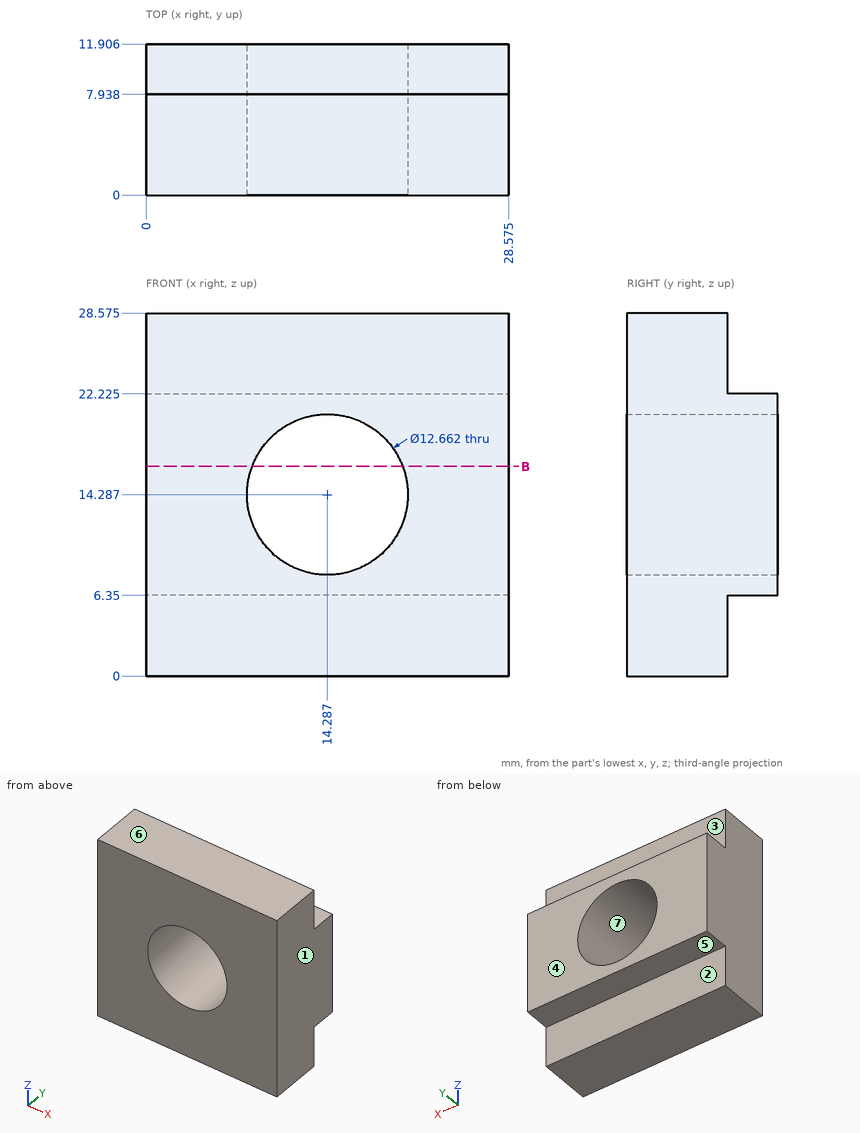
Can you work these out from the drawing? Everything is in mm from the part's minimum corner. A direction names the side the tool comes from. Give positions to 0.01 mm unless a question says otherwise; leave off trailing zeros. Order: outer loops, then holes, each group sorted by start corner. A loop starts at its lowest first (then second) coordinate and runs counter-clockwise, first axis right, second up. Notation, with made-up numbers: M 65.5,50.5 L 71.5,50.5 A30 ccw 71.5,87.5 Z; hole C 87,24.25 d4. An arc over 180 degrees is marked long. Use a Markdown table: item, result. Add a question column.
1. I need wall thicknesses on probe 1 along Y at (x, z) = (11.5, 2.5); probe 2 along X at (y, z) = (5.75, 12.5) (1 decimal); probe 3 along Z at (x, y) = (13.25, 6) (1 decimal). Which ranges of each line are inside material? Lowest first, please. Write a range as from..to.
2. If we mould it in two halves opening along Z, with no side actions, what happens to the marked faces 4, 5, 6 and 7? For each: +Z half, -Z half, draft (parallel to the pull), parting line (faces both ways), or undercut.
3. On a 3-axis mill with a long thin cutter (end or side, diameter ignored), from which of +Z, -Z, +X, -X, +Y, -Y can I reach the whole of each face in a straight line? I mean the marked faces 1, 2 and 3. Say none if no direction works.
4. For pin 1 Ø3 at (x, y) = (13, 10) entering from -Z; pin 2 Ø7 at (x, z) = (9, 2) entering from +Y; pin 3 Ø7.5 at (x, z) = (14.29, 14.29) entering from -Y, each with a flat end and sliding along its axis, tell me the tip position at first contact or that it passes through.
5. Suppose I cut it at B-B (z = 16.5). List the corners of the cut face in (x, y) for me (1 decimal).
Results list:
| question | item | result |
|---|---|---|
| 1 | probe 1 | y = 0..7.94 |
| 1 | probe 2 | x = 0..8.2, 20.4..28.6 |
| 1 | probe 3 | z = 0..8, 20.5..28.6 |
| 2 | face 4 | draft |
| 2 | face 5 | -Z half |
| 2 | face 6 | +Z half |
| 2 | face 7 | undercut |
| 3 | face 1 | +Z, -Z, +X, +Y, -Y |
| 3 | face 2 | -Z, +X, -X, +Y |
| 3 | face 3 | +Z, +X, -X, +Y |
| 4 | pin 1 | stops at z = 6.35 |
| 4 | pin 2 | stops at y = 7.94 |
| 4 | pin 3 | passes through |
| 5 | outline | M 0,0 L 8.4,0 L 8.4,11.9 L 0,11.9 Z; M 20.2,0 L 28.6,0 L 28.6,11.9 L 20.2,11.9 Z |
